Build history of the part. All positions in model axes, mm. Face numbers are marked on the shaded views. A direction names the side the tool comes from. Give positions to 0.01 mm unless a question says otherwise; leave off trailing zeros. Order: outer loops, then holes, each group sorted by start corner. A loop starts at its lowest first (then second) coordinate and runs counter-clockwise, first axis right, second up. Notation, with made-up numbers: (65, -1.5) -> (88, -1.5) arc R13 ccw to (88, 5.5) -> close; hole circle Ø8 at (5, 41). An arc over 180 degrees is marked (long way). One line per item, written item: value. Start each with the question number.
(1) Saw through at C-C on z = 2.5. Give the cut face in (x, y), plus the area to 3 significant figures.
(2) Which spindle directions (+Z, -Z, +X, -X, +Y, -Y) get a long thin tool onto all of the face, cutting with end or side? Do the marked faces 4 and 5. Say none if no direction does.
(3) Saw through at D-D on x = 1.65. Give the cut face in (y, z).
(4) Saw through at B-B on y = 0.85. Give the cut face in (x, z).
(5) Pin check, flat tips, straight feed: pin 1 (3 mm diameter, centred on x = -1, z = 5.5, fed in from -Y); pin 2 (1.5 mm diameter, centred on x = 0, y = 0, fed in from -Z); pin 3 (3 mm diameter, centred on x = 0, y = -0.5, fed in from -Z). Stop position of each tip, or through.
(6) Two-plate mould, pull along X, no slides. Class the marked faces 1, 2 and 3: +X half, -X half, draft (parallel to the pull), parting line (faces both ways), or undercut.
(7) Probe line 1 (Y direction, x = 0, z = -2.65); line 2 (Z direction, x = 0, y = 0.7); line 3 (Z direction, x = -0.2, y = 1.85). List the from-to ranges inside material, lowest first.
(8) Saw through at A-A on x = 0. Give the cut face in (y, z), plus the area to 3 significant figures.
Autodesk Inventor part; units mm, degrees
ref_plane "Work Plane1" through (0, 0, -3) normal (0, 0, 1) x (1, 0, 0)
ref_plane "Work Plane2" through (0, 0, 3.0398) normal (0, 0, 1) x (1, 0, 0)
ref_plane "Work Plane3" through (0, 0, -3) normal (0, 0, 1) x (1, 0, 0)
ref_plane "Work Plane1" through (0, 0, -3) normal (0, 0, 1) x (1, 0, 0)
sketch "Sketch1" plane through (0, 0, -3) normal (0, 0, 1) x (1, 0, 0)
  circle A0 centre (0, 0) radius 2.75
extrude "M3_Head_Envelope" add sketch "Sketch1" along normal blind 3
sketch "Sketch2" plane through (0, 0, 0) normal (0, 0, 1) x (1, 0, 0)
  circle A0 centre (0, 0) radius 1.5
extrude "M3_Clearance_Grip" add sketch "Sketch2" along normal blind 3.0398
ref_plane "Work Plane2" through (0, 0, 3.0398) normal (0, 0, 1) x (1, 0, 0)
sketch "Sketch3" plane through (0, 0, 3.0398) normal (0, 0, 1) x (1, 0, 0)
  circle A0 centre (0, 0) radius 1.25
extrude "Thread_Core_No_Helix" add sketch "Sketch3" along normal blind 4.9602
ref_plane "Work Plane3" through (0, 0, -3) normal (0, 0, 1) x (1, 0, 0)
sketch "Sketch4" plane through (0, 0, -3) normal (0, 0, 1) x (1, 0, 0)
  circle A0 centre (0, 0) radius 1.25
extrude "Extrusion4" cut sketch "Sketch4" along normal blind 1.5
properties part number "Device_M3x8_Simplified"
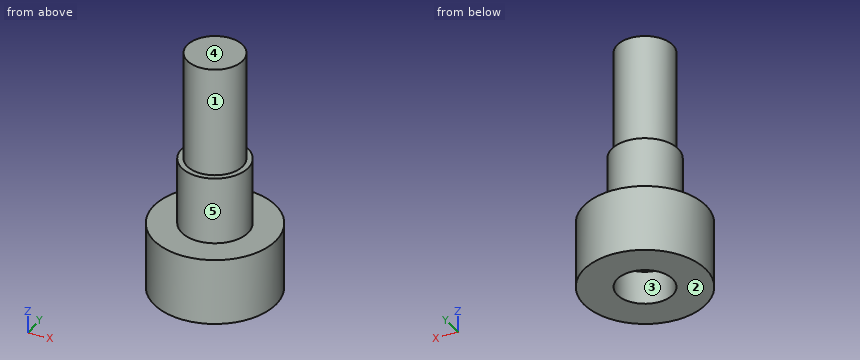
Results below:
1. outline: circle Ø3 at (0, 0)
1. area: 7.07 mm²
2. face 4: +Z, +X, -X, +Y, -Y
2. face 5: +Z
3. outline: (-2.2, -3) -> (2.2, -3) -> (2.2, 0) -> (-2.2, 0) -> close
4. outline: (-2.62, -3) -> (-0.92, -3) -> (-0.92, -1.5) -> (0.92, -1.5) -> (0.92, -3) -> (2.62, -3) -> (2.62, 0) -> (1.24, 0) -> (1.24, 3.04) -> (0.92, 3.04) -> (0.92, 8) -> (-0.92, 8) -> (-0.92, 3.04) -> (-1.24, 3.04) -> (-1.24, 0) -> (-2.62, 0) -> close
5. pin 1: stops at y = -1.25
5. pin 2: stops at z = -1.5
5. pin 3: stops at z = -3
6. face 1: parting line
6. face 2: draft
6. face 3: undercut
7. line 1: y = -2.75 to -1.25, 1.25 to 2.75
7. line 2: z = -1.5 to 8
7. line 3: z = -3 to 0
8. outline: (-2.75, -3) -> (-1.25, -3) -> (-1.25, -1.5) -> (1.25, -1.5) -> (1.25, -3) -> (2.75, -3) -> (2.75, 0) -> (1.5, 0) -> (1.5, 3.04) -> (1.25, 3.04) -> (1.25, 8) -> (-1.25, 8) -> (-1.25, 3.04) -> (-1.5, 3.04) -> (-1.5, 0) -> (-2.75, 0) -> close
8. area: 34.3 mm²
